Autodesk Inventor part; units mm, degrees
ref_plane "YZ Plane" through (0, 0, 0) normal (1, 0, 0) x (0, 1, 0)
ref_plane "XZ Plane" through (0, 0, 0) normal (0, 1, 0) x (-1, 0, 0)
ref_plane "XY Plane" through (0, 0, 0) normal (0, 0, 1) x (1, 0, 0)
sketch "Sketch1" plane through (0, 0, 0) normal (0, 0, 1) x (1, 0, 0)
  line L0 (0, 9) -> (2.75, 9)
  line L1 (2.75, 9) -> (2.75, 6)
  line L2 (2.75, 6) -> (1.5, 6)
  line L3 (1.5, 6) -> (1.5, 0)
  line L4 (1.5, 0) -> (0, 0)
  line L5 (0, 0) -> (0, 9)
  dimension "d0" = 2.75
  dimension "d1" = 3
  dimension "d2" = 6
  dimension "d3" = 1.5
revolve "Revolution1" add sketch "Sketch1" angle 360 about axis through (0, 0, 0) along (0, 1, 0)
thread "Thread1"
sketch "Sketch3" plane through (0, 9, 0) normal (0, 1, 0) x (1, 0, 0)
  line L0 (1.25, -0.7217) -> (0, -1.4434)
  line L1 (0, -1.4434) -> (-1.25, -0.7217)
  line L2 (-1.25, -0.7217) -> (-1.25, 0.7217)
  line L3 (-1.25, 0.7217) -> (0, 1.4434)
  line L4 (0, 1.4434) -> (1.25, 0.7217)
  line L5 (1.25, 0.7217) -> (1.25, -0.7217)
  point P0 (0, 0)
  point P1 (0, 0)
  dimension "d13" = 2.5
extrude "Extrusion2" cut sketch "Sketch3" against normal blind 1.5
chamfer "Chamfer2" distance 0.1 angle 45 16 edges at (0.625, 9, 1.0825) (1.25, 9, 0) (1.25, 7.5, 0) (0.625, 9, -1.0825) (0.625, 7.5, -1.0825) (-0.625, 9, -1.0825) (-0.625, 7.5, -1.0825) (-1.25, 7.5, 0) (-1.25, 9, 0) (-0.625, 7.5, 1.0825) (-0.625, 9, 1.0825) (0.625, 7.5, 1.0825) (-2.75, 9, 0) (-2.75, 6, 0) (-1.5, 6, 0) (-1.5, 0, 0)
properties part number "M3 X 6"
Could you check a few things on this model? Use its own coordinates, in mm. A direction names the side the tool comes from. Round coordinates to 2 decimals unless told otherwise and drop trailing zeros. Loops run counter-clockwise (first coordinate to the right, second up) from the corner with the lowest first, then second, coordinate; pieces in that order, holes last. Notation, with made-up numbers: (-16.75, -7.5) -> (12.25, -7.5) arc R20 cw to (12.25, 8.5) -> close; hole circle Ø4 at (80.5, 62.25). An arc over 180 degrees is marked (long way). Put each result on its own line as item: value.
Q1. I want a section at A-A on z = 0. Write out the boundary of the cut face in (x, y), and give its area (3 significant figures).
Checks:
outline: (-2.75, 6.1) -> (-2.65, 6) -> (-1.6, 6) -> (-1.5, 5.9) -> (-1.5, 0.1) -> (-1.4, 0) -> (1.4, 0) -> (1.5, 0.1) -> (1.5, 5.9) -> (1.6, 6) -> (2.65, 6) -> (2.75, 6.1) -> (2.75, 8.9) -> (2.65, 9) -> (1.35, 9) -> (1.25, 8.9) -> (1.25, 7.6) -> (1.15, 7.5) -> (-1.15, 7.5) -> (-1.25, 7.6) -> (-1.25, 8.9) -> (-1.35, 9) -> (-2.65, 9) -> (-2.75, 8.9) -> close
area: 30.7 mm2
Q2. Which directions (+Z, -Z, +X, -X, +Y, -Y) give clear straight access to the entire face, cutting with the end or side of a thin tool? Please do faces 4 (the flat face through (1.1, 9, 1.1)), 5 (the flat face through (-0.616, 8.259, 1.088)), 6 (the flat face through (0, 6, 2)).
Checks:
face 4: +Z, -Z, +X, -X, +Y
face 5: +Y
face 6: -Y
Q3. For pin 1 Ø1.5 at (y, z) = (7, 0.5) entering from -X; pin 2 Ø1.5 at (x, y) = (1, 2.5) entering from -Z; pin 3 Ø2 at (x, y) = (1.5, 7.5) entering from -Z; pin 4 Ø0.7 at (x, z) = (0, -0.5) entering from +Y, each with a flat end and sliding along its axis, tell me the tip position at first contact or that it passes through.
Checks:
pin 1: x = -2.75
pin 2: z = -1.48
pin 3: z = -2.7
pin 4: y = 7.5
Q4. I want a section at B-B on y = 5.25. Write out the boundary of the cut face in (x, z), and give its area (3 significant figures).
Checks:
outline: circle Ø3 at (0, 0)
area: 7.07 mm2
Q5. Please list where these lines run through material, in increasing order: line 1 (Y direction, x = 0.2, z = -1.05); line 2 (Y direction, x = -1.8, z = 0.95); line 3 (Z direction, x = 0.7, y = 7.75). Write a range as from..to.
Checks:
line 1: 0..7.5
line 2: 6..9
line 3: -2.66..-1.04, 1.04..2.66
Q6. Thinking about a two-plate mould opening in X: for faces 1 (the flat face through (0, 0, 0)), 2 (the flat face through (0.616, 8.259, -1.088)), 3 (the cylindrical face through (-1.5, 2.96, 0.07)), which applies, pulls with the +X half, pulls with the -X half, needs draft (parallel to the pull), parting line crosses it, or undercut?
Checks:
face 1: needs draft
face 2: undercut
face 3: parting line crosses it
